Source: three-view drawing plus pictorial views. Frame: mm from the lowest corner of the part. Coordinates: 2 decimals unless noted, no trailing zeros. Loops run counter-clockwise (first coordinate to the right, second up) from the corner with the lowest first, then second, coordinate; pieces in that order, holes last. Notation, with made-up numbers: (52.5, 59.25) - (78.5, 59.25) arc R15 ccw to (78.5, 78.25) - close; hole circle Ø8 at (-10, 42.5). An arc over 180 degrees is marked (long way). Use CSV: the item, a comma, the result in double quotes. Start each with the question number.
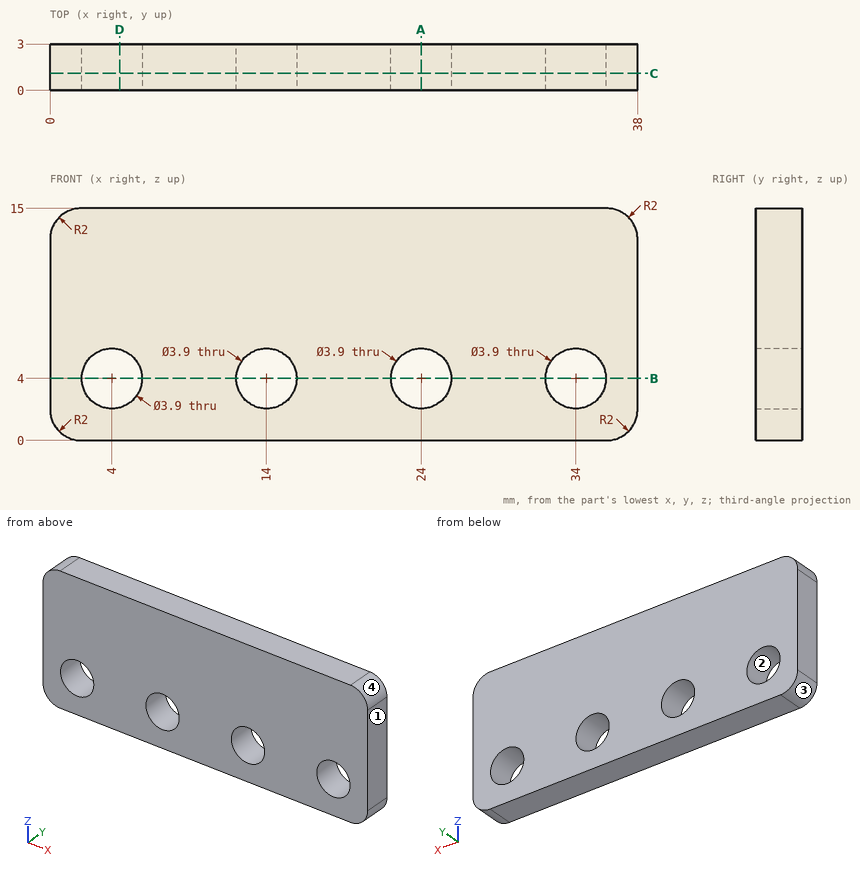
(1) Section A-A on x = 24. Output: boundary loops of the cut face in (y, z), plus the area to 3 significant figures.
(2) Draft query along Z for the marked faces 1, 2, 3 and 4. Return one class per face: released by +Z, released by -Z, zero draft, split by the parting line, or undercut.
(3) Section B-B on z = 4. Output: boundary loops of the cut face in (x, y), plus the area to 3 significant figures.
(4) Section D-D on x = 4.5. Output: boundary loops of the cut face in (y, z), plus the area to 3 significant figures.
(5) Section C-C on y = 1.1. Output: boundary loops of the cut face in (x, z).
(6) Pin query (flat end, axial travel): pin 1 Ø3 at (x, z) = (14, 4) entering from -Y. Return the tip coordinate at first contact, or that it passes through.
(7) Ray query, line 1 (X direction, y = 1.8, z = 4); line 2 (X direction, y = 2.45, z = 5); line 3 (Z direction, x = 24.5, y = 1.45). Return the intervals inside material, ascending. Write a range as [from, to].
Solution:
1,outline,"(0, 0) - (3, 0) - (3, 2.05) - (0, 2.05) - close; (0, 5.95) - (3, 5.95) - (3, 15) - (0, 15) - close"
1,area,"33.3 mm²"
2,face 1,"zero draft"
2,face 2,"undercut"
2,face 3,"released by -Z"
2,face 4,"released by +Z"
3,outline,"(0, 0) - (2.05, 0) - (2.05, 3) - (0, 3) - close; (5.95, 0) - (12.05, 0) - (12.05, 3) - (5.95, 3) - close; (15.95, 0) - (22.05, 0) - (22.05, 3) - (15.95, 3) - close; (25.95, 0) - (32.05, 0) - (32.05, 3) - (25.95, 3) - close; (35.95, 0) - (38, 0) - (38, 3) - (35.95, 3) - close"
3,area,"67.2 mm²"
4,outline,"(0, 0) - (3, 0) - (3, 2.12) - (0, 2.12) - close; (0, 5.88) - (3, 5.88) - (3, 15) - (0, 15) - close"
4,area,"33.7 mm²"
5,outline,"(0, 2) arc R2 ccw to (2, 0) - (36, 0) arc R2 ccw to (38, 2) - (38, 13) arc R2 ccw to (36, 15) - (2, 15) arc R2 ccw to (0, 13) - close; hole circle Ø3.9 at (4, 4); hole circle Ø3.9 at (14, 4); hole circle Ø3.9 at (24, 4); hole circle Ø3.9 at (34, 4)"
6,pin 1,"passes through"
7,line 1,"x = [0, 2.05], [5.95, 12.05], [15.95, 22.05], [25.95, 32.05], [35.95, 38]"
7,line 2,"x = [0, 2.33], [5.67, 12.33], [15.67, 22.33], [25.67, 32.33], [35.67, 38]"
7,line 3,"z = [0, 2.12], [5.88, 15]"
